Source: CAD feature listing. Evaluate the final solid. Frame: model axes, mm. A direction names the side the tool comes from. Give positions to 0.01 mm unless a question says otherwise; leave off trailing zeros. Write each loop counter-clockwise with the first axis right and the second up, starting at its lowest first coordinate (ties: lowest second). Pieces come first, ordered by that corner, then holes. Notation, with made-up numbers: (22, 44) -> (68, 44) arc R24 ccw to (68, 54) -> close; hole circle Ø5 at (-24.75, -27). An arc over 180 degrees is marked (long way). Write item = value, one per line.
from build123d import *
from build123d.topology import SkipClean

# Parameters (mm, degrees)
BOSS_EXTRUDE1_DEPTH      = 60
SKETCH3_R                = 6.000000000000003
SKETCH3_R_2              = 5.999999999999998
CUT_EXTRUDE1_DEPTH       = 10
SKETCH4_R                = 3.0000000000000027
SKETCH4_R_2              = 3.0000000000000004
SKETCH4_R_3              = 2.9999999999999996
CUT_EXTRUDE2_DEPTH       = 7
BOSS_EXTRUDE2_DEPTH      = 40
BOSS_EXTRUDE2_DEPTH_BACK = 20
CUT_EXTRUDE3_DEPTH       = 90.70884954089212
CUT_EXTRUDE3_DEPTH_BACK  = 40
BOSS_EXTRUDE3_DEPTH      = 10
CUT_EXTRUDE4_START       = -60
SKETCH9_R                = 10.999999999999993
CUT_EXTRUDE4_DEPTH       = 60
CUT_EXTRUDE5_DEPTH       = 60
SKETCH9_4_W              = 6
SKETCH9_4_H              = 24.979661142970425
CUT_EXTRUDE6_DEPTH       = 7


with BuildPart() as part:
    # Sketch2 → Boss-Extrude1 (new body)
    with BuildSketch(Plane.XY):
        Polygon((-32.63636363636363, -18.753246753246753), (-32.63636363636363, 11.246753246753245), (-18.636363636363633, 11.246753246753245), (-18.636363636363633, 8.246753246753245), (-2.6363636363636314, 8.246753246753245), (-2.6363636363636314, 11.246753246753245), (37.363636363636374, 11.246753246753245), (37.363636363636374, 1.2467532467532443), (-22.636363636363637, 1.2467532467532365), (-22.63636363636363, -18.75324675324675), align=None)
    extrude(amount=BOSS_EXTRUDE1_DEPTH)

    # Sketch3 → Cut-Extrude1 (cut)
    with BuildSketch(Plane.ZY.offset(32.63636363636363)):
        with Locations((45, -8.753246753246755)):
            Circle(SKETCH3_R)
        with Locations((15, -8.753246753246755)):
            Circle(SKETCH3_R_2)
    extrude(amount=-CUT_EXTRUDE1_DEPTH, mode=Mode.SUBTRACT)

    # Sketch4 → Cut-Extrude2 (cut)
    with BuildSketch(Plane(origin=(0, 8.246753246753245, 0), x_dir=(1, 0, 0), z_dir=(0, 1, 0))):
        with Locations(Location((-10.63636363636363, -49.99999999999999, 0), (0, 0, 270))):
            Circle(SKETCH4_R)
        with Locations(Location((-10.636363636363631, -9.999999999999995, 0), (0, 0, 270))):
            Circle(SKETCH4_R_2)
        with Locations(Location((-10.63636363636363, -29.999999999999996, 0), (0, 0, 270))):
            Circle(SKETCH4_R_3)
    extrude(amount=-CUT_EXTRUDE2_DEPTH, mode=Mode.SUBTRACT)

    # Sketch5 → Boss-Extrude2 (add, two sides: drawn at the far end of the back side and taken through both)
    with BuildSketch(Plane(origin=(0, 11.246753246753245, 0), x_dir=(1, 0, 0), z_dir=(0, 1, 0)).offset(-BOSS_EXTRUDE2_DEPTH_BACK)):
        with BuildLine():
            ThreePointArc((37.36363636363612, -46), (40.532227080018274, -45.6831129841004), (43.57530713931024, -44.745004109007205))
            ThreePointArc((43.57530713931024, -44.745004109007205), (50.693803887167014, -38.849103558813695), (53.363636363636374, -30.000000000000004))
            ThreePointArc((53.363636363636374, -30), (50.693803887167014, -21.150896441186312), (43.57530713931025, -15.254995890992799))
            ThreePointArc((43.57530713931025, -15.254995890992799), (40.53222708001828, -14.316887015899601), (37.36363636363611, -13.999999999999996))
            Line((37.363636363636374, -14), (37.363636363636374, -19.000000000000007))
            ThreePointArc((37.36363636363639, -19.000000000000007), (45.141810956688396, -22.22182540694799), (48.36363636363637, -30))
            ThreePointArc((48.36363636363637, -30.000000000000004), (45.14181095668839, -37.77817459305202), (37.363636363636374, -40.99999999999999))
            Line((37.363636363636374, -40.99999999999999), (37.363636363636374, -46))
        make_face()
        with BuildLine():
            ThreePointArc((37.36363636363611, -13.999999999999996), (21.36363636363637, -29.999999999999996), (37.36363636363612, -46))
            Line((37.363636363636374, -46), (37.363636363636374, -40.99999999999999))
            ThreePointArc((37.363636363636374, -40.99999999999999), (26.36363636363638, -29.99999999999999), (37.36363636363639, -19.000000000000007))
            Line((37.363636363636374, -19.000000000000007), (37.363636363636374, -14))
        make_face()
    extrude(amount=BOSS_EXTRUDE2_DEPTH + BOSS_EXTRUDE2_DEPTH_BACK)

    # Sketch5<4> → Cut-Extrude3 (cut, two sides: drawn at the far end of the back side and taken through both)
    with BuildSketch(Plane(origin=(0, 11.246753246753245, 0), x_dir=(1, 0, 0), z_dir=(0, 1, 0)).offset(-CUT_EXTRUDE3_DEPTH_BACK)):
        Polygon((7.363636363636369, 0), (37.36363636363637, -12.638187272961233), (37.363636363636374, 0), align=None)
        Polygon((37.363636363636374, -47.36181272703875), (7.36363636363637, -60), (37.363636363636374, -60), align=None)
    extrude(amount=CUT_EXTRUDE3_DEPTH + CUT_EXTRUDE3_DEPTH_BACK, mode=Mode.SUBTRACT)

    # Sketch7 → Boss-Extrude3 (add)
    with BuildSketch(Plane(origin=(0, 11.246753246753245, 0), x_dir=(1, 0, 0), z_dir=(0, 1, 0))):
        Polygon((37.363636363636374, -12.638187272961241), (43.57530713931025, -15.254995890992793), (43.57530713931024, -44.7450041090072), (37.363636363636374, -47.361812727038746), align=None)
    extrude(amount=-BOSS_EXTRUDE3_DEPTH)

    # Sketch9 → Cut-Extrude4 (cut)
    with SkipClean():  # the faces are left unmerged after this step: merging them gives an invalid solid
        with BuildSketch(Plane(origin=(0, 51.24675324675325, 0), x_dir=(1, 0, 0), z_dir=(0, 1, 0)).offset(CUT_EXTRUDE4_START)):
            with Locations(Location((37.363636363636374, -30, 0), (0, 0, 270))):
                Circle(SKETCH9_R)
        extrude(amount=CUT_EXTRUDE4_DEPTH, mode=Mode.SUBTRACT)

    # Sketch9<3> → Cut-Extrude5 (cut)
    with BuildSketch(Plane(origin=(0, 51.24675324675325, 0), x_dir=(1, 0, 0), z_dir=(0, 1, 0))):
        Polygon((49.86363636363637, -27), (49.86363636363636, -33), (47.38496613189031, -32.99999999999999), (47.38496613189031, -27), align=None)
    extrude(amount=-CUT_EXTRUDE5_DEPTH, mode=Mode.SUBTRACT)

    # Sketch9<4> → Cut-Extrude6 (cut)
    with BuildSketch(Plane(origin=(0, 51.24675324675325, 0), x_dir=(1, 0, 0), z_dir=(0, 1, 0))):
        with Locations((37.363636363636374, -17.510169428514793)):
            Rectangle(SKETCH9_4_W, SKETCH9_4_H)
    extrude(amount=-CUT_EXTRUDE6_DEPTH, mode=Mode.SUBTRACT)


solid = part.part
1) Cut plane D-D (x = 2). Return the cut outline in (y, z), then the cut area to 3 significant figures.
Computed:
outline = (1.25, 0) -> (11.25, 0) -> (11.25, 60) -> (1.25, 60) -> close
area = 600 mm²
2) Access query for faces 1 (the cylindrical face through (-27.706, -8.489, 39.006)), 2 (the flat face through (-26, 11.247, 30)), 3 (the flat face through (40.364, 48, 17)). Directions: +Z, -Z, +X, -X, +Y, -Y. A direction counts if a zero-diameter tool reaches every point of the face in a straight line with its end or side. Return the directions, or none.
Computed:
face_1 = -X
face_2 = +Z, -Z, -X, +Y
face_3 = -Z, +Y
3) Cut plane C-C (z = 17.5). Return the cut outline in (x, y), then the cut area to 3 significant figures.
Computed:
outline = (-32.64, -18.75) -> (-22.64, -18.75) -> (-22.64, -14.21) -> (-32.64, -14.21) -> close; (-32.64, -3.3) -> (-22.64, -3.3) -> (-22.64, 1.25) -> (27.38, 1.25) -> (27.38, -8.75) -> (47.35, -8.75) -> (47.35, 51.25) -> (40.36, 51.25) -> (40.36, 44.25) -> (34.36, 44.25) -> (34.36, 51.25) -> (27.38, 51.25) -> (27.38, 11.25) -> (-2.64, 11.25) -> (-2.64, 8.25) -> (-18.64, 8.25) -> (-18.64, 11.25) -> (-32.64, 11.25) -> close
area = 1,800 mm²
4) Cut plane B-B (y = 47.5). Return the cut outline in (x, z), then the cut area to 3 significant figures.
Computed:
outline = (34.36, 14.28) -> (34.36, 19.42) arc R11 cw (long way) to (47.95, 33) -> (49.86, 33) -> (49.86, 27) -> (47.95, 27) arc R11 cw to (40.36, 19.42) -> (40.36, 14.28) arc R16 ccw (long way) to start
area = 384 mm²
5) Material intervals for L1, parallel to Y at x = -28.75, z = 15; L2, parallel to Y at x = 23, z = 51; L3, parallel to X at y = 38, z = 37.5, sorted ascending.
Computed:
L1 = -18.75 to -14.75, -2.75 to 11.25
L2 = 1.25 to 11.25
L3 = 23.23 to 29.32, 45.41 to 51.5
6) Contact query for flat-ended pins moving along their axis: pin 1 (1.8 mm diameter, centred on y = 32.5, z = 29.5, fed in from -X); pin 2 (0.6 mm diameter, centred on x = 49, y = 34, fed in from +Z); pin 3 (5.5 mm diameter, centred on y = 49, z = 15.5, fed in from -X); pin 4 (5 mm diameter, centred on x = -10.64, z = 10, fed in from +Y). Output: stop coordinate, or through.
Computed:
pin_1 = 21.36
pin_2 = 41.29
pin_3 = 26.5
pin_4 = through
7) Cut plane A-A (z = 30). Return the cut outline in (x, y), then the cut area to 3 significant figures.
Computed:
outline = (-32.64, -18.75) -> (-22.64, -18.75) -> (-22.64, 1.25) -> (-13.64, 1.25) -> (-13.64, 8.25) -> (-18.64, 8.25) -> (-18.64, 11.25) -> (-32.64, 11.25) -> close; (-7.64, 1.25) -> (21.36, 1.25) -> (21.36, -8.75) -> (26.36, -8.75) -> (26.36, 51.25) -> (21.36, 51.25) -> (21.36, 11.25) -> (-2.64, 11.25) -> (-2.64, 8.25) -> (-7.64, 8.25) -> close; (49.86, -8.75) -> (53.36, -8.75) -> (53.36, 51.25) -> (49.86, 51.25) -> close
area = 1,160 mm²
8) Draft query along X for faces 4 (the flat face through (11, 11.247, 30)), 5 (the flat face through (-32.636, -4, 30)), 6 (the cylindrical face through (-10.504, 4.796, 27.003)). Return one class per face: pulls with the +X half, pulls with the -X half, needs draft (parallel to the pull), parting line crosses it, or undercut.
Computed:
face_4 = needs draft
face_5 = pulls with the -X half
face_6 = undercut
